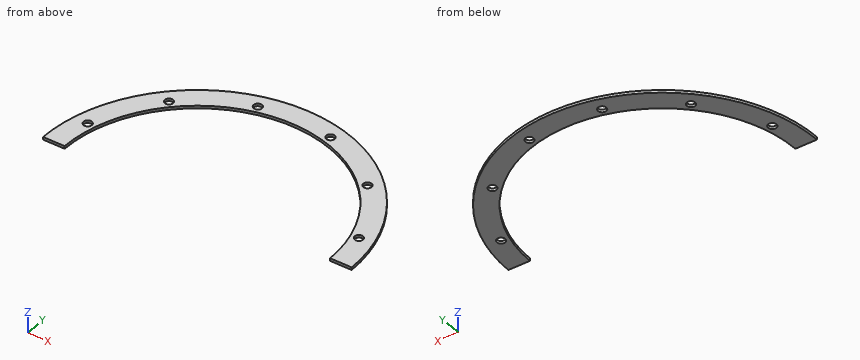
from build123d import *

# Parameters (mm, degrees)
BOSS_EXTRUDE1_DEPTH   = 1.5875
F_8_CLEARANCE_HOLE1_D = 4.9149
CIRPATTERN1_COUNT     = 6
CIRPATTERN1_ANGLE     = 150


with BuildPart() as part:
    # Sketch1 → Boss-Extrude1 (new body)
    with BuildSketch(Plane.XY):
        with BuildLine():
            Line((-90.7, 0), (-78, 0))
            ThreePointArc((-78, 0), (0, 78), (78, 0))
            Line((78, 0), (90.7, 0))
            ThreePointArc((90.7, 0), (0, 90.7), (-90.7, 0))
        make_face()
    extrude(amount=BOSS_EXTRUDE1_DEPTH)

    # #8 Clearance Hole1 (through all)
    with Locations(Plane.XY.offset(1.5875)):
        with Locations((79.688880669, 21.352571221)):
            f_8_clearance_hole1 = Hole(F_8_CLEARANCE_HOLE1_D / 2)

    # CirPattern1: #8 Clearance Hole1 ×6 about axis
    cirpattern1_axis = Axis((0, 0, 0), (0, 0, 1))
    for i in range(1, CIRPATTERN1_COUNT):
        add(f_8_clearance_hole1.rotate(cirpattern1_axis, i * CIRPATTERN1_ANGLE / (CIRPATTERN1_COUNT - 1)), mode=Mode.SUBTRACT)


solid = part.part
The model under review builds one solid part; all positions refer to its coordinate system, in mm. Give positions to 0.01 mm unless a question says otherwise; leave off trailing zeros. Order: outer loops, then holes, each group sorted by start corner. A loop starts at its lowest first (then second) coordinate and runs counter-clockwise, first axis right, second up. Notation, with made-up numbers: M 14.5,24 L 31.5,24 A6 ccw 31.5,29 Z; hole C 85,6 d6. An arc over 180 degrees is marked long. Use one line per item in the form item = value. Start each with the question number.
Item 1: Insertion check: pin 1 Ø4.5 at (x, y) = (-58.34, 58.34) entering from -Z; pin 2 Ø6.5 at (x, y) = (58.34, 58.34) entering from +Z. Each pin has a flat end and moves straight along its axis. Give the tip position at first contact, or say it passes through.
Item 2: We need section C-C on z = 0.3. Give the boundary of the cut face in (x, y), plus the area to 3 significant figures.
Item 3: We need section A-A on y = 35. Give the boundary of the cut face in (x, z).
Item 4: We need section B-B on y = 59. Give the boundary of the cut face in (x, z).
Item 5: We need section D-D on x = 0. Give the boundary of the cut face in (y, z).
Item 6: To check wall thickness, follow line 1 along X through (y, z) = (22.5, 0.3); line 2 along X through (y, z) = (80.5, 0.95); line 3 along X through (y, z) = (14.5, 0.35). State the ranges of each line that lie inside material, in increasing order. Write a range as from..to.
Completed:
q1.pin_1 = through
q1.pin_2 = 1.59
q2.outline = M -90.7,0 L -78,0 A78 cw 78,0 L 90.7,0 A90.7 ccw Z; hole C -79.69,21.35 d4.91; hole C -58.34,58.34 d4.91; hole C -21.35,79.69 d4.91; hole C 21.35,79.69 d4.91; hole C 58.34,58.34 d4.91; hole C 79.69,21.35 d4.91
q2.area = 3,250 mm²
q3.outline = M -83.67,0 L -69.71,0 L -69.71,1.59 L -83.67,1.59 Z; M 69.71,0 L 83.67,0 L 83.67,1.59 L 69.71,1.59 Z
q4.outline = M -68.89,0 L -60.7,0 L -60.7,1.59 L -68.89,1.59 Z; M -55.97,0 L -51.02,0 L -51.02,1.59 L -55.97,1.59 Z; M 51.02,0 L 55.97,0 L 55.97,1.59 L 51.02,1.59 Z; M 60.7,0 L 68.89,0 L 68.89,1.59 L 60.7,1.59 Z
q5.outline = M 78,0 L 90.7,0 L 90.7,1.59 L 78,1.59 Z
q6.line_1 = -87.86..-81.86, -77.52..-74.68, 74.68..77.52, 81.86..87.86
q6.line_2 = -41.79..-23.67, -19.03..19.03, 23.67..41.79
q6.line_3 = -89.53..-76.64, 76.64..89.53
